Could you check a few things on this model? Use its own coordinates, in mm. A direction names the side the tool comes from. Give positions to 0.01 mm unless a question says otherwise; leave off trailing zeros. Order: outer loops, then holes, each group sorted by start corner. A loop starts at its lowest first (then second) coordinate and runs counter-clockwise, first axis right, second up.
(1) Imagine slicing it at C-C, the plane y = 37. Write out the boundary of the cut face in (x, z), then the cut area to 3 significant figures.
(2) If I drill on probe 1 along X at (y, z) = (2.7, 11.5); probe 2 along Y at (x, z) = (11, 6); probe 3 along Y at (x, z) = (-0.75, -5.5), over which ranges is the centre line in solid material (lowest first)?
(3) Imagine slicing it at A-A, the plane z = 0. Write out the boundary of the cut face in (x, y) (3 decimals), then the cut area to 3 significant figures.
(4) On a 3-axis mill with a long thin cutter (end or side, diameter ignored), from which of +Z, -Z, +X, -X, +Y, -Y can I reach the whole of each face in a straight line? I mean faces 5 (the flat face through (-11, 5, 12)), 6 (the flat face through (8.5, 30, -12)), 7 (the flat face through (-8.5, 30, 12)), 8 (the cylindrical face through (9.1, 30.06, 9.07)). Say none if no direction works.
(5) If we mould it in two halves opening along Z, with no side actions, what happens to faces 1 (the flat face through (-11, 5, -11)), 2 (the cylindrical face through (1.01, 14.28, 0.65)), 3 (the flat face through (14, 16, 0)), 4 (the flat face through (-12, 30, 8.5))? For each: released by +Z, released by -Z, zero draft, split by the parting line, or undercut.
(6) Imagine slicing it at B-B, the plane x = 0. Write out the boundary of the cut face in (y, z) (3 decimals), then the cut area to 3 significant figures.
(7) Will these pins go through, and if not, where does the flat tip stop? pin 1 (0.8 mm diameter, centred on y = 30, z = 12, fed in from +X); pin 2 (2.5 mm diameter, centred on x = -10, z = -11.5, fed in from +Y); pin 3 (5.5 mm diameter, centred on x = 10, z = 10, fed in from +Y).
(8) Imagine slicing it at D-D, the plane x = -4. Write out the boundary of the cut face in (y, z), then the cut area to 3 significant figures.
from build123d import *

# Parameters (mm, degrees)
SKETCH_1_W          = 28
SKETCH_1_H          = 28
EXTRUDE_1_DEPTH     = 31.8
SKETCH_2_R          = 10.975
EXTRUDE_2_DEPTH     = 2
SKETCH_3_R          = 2.5
EXTRUDE_3_DEPTH     = 18.2
EXTRUDE_START       = 16
SKETCH_4_R          = 2.5
EXTRUDE_4_DEPTH     = 16
FILLET_1_R          = 2
SKETCH_5_R          = 1.25
CUT_EXTRUDE_1_DEPTH = 5
CUT_EXTRUDE_2_DEPTH = 2.5
CHAMFER_1_SIZE      = 1
FILLET_2_R          = 0.5
SKETCH_7_R          = 1.2
CUT_EXTRUDE_3_DEPTH = 71.823724858


with BuildPart() as part:
    # 草图1 → 凸台-拉伸1 (new body)
    with BuildSketch(Plane(origin=(0, 0, 0), x_dir=(1, 0, 0), z_dir=(0, 1, 0))):
        Rectangle(SKETCH_1_W, SKETCH_1_H)
    extrude(amount=EXTRUDE_1_DEPTH)

    # 草图2 → 凸台-拉伸2 (add)
    with BuildSketch(Plane(origin=(0, 0, 0), x_dir=(-1, 0, 0), z_dir=(0, -1, 0))):
        with Locations(Location((0, 0, 0), (0, 0, 90))):
            Circle(SKETCH_2_R)
    extrude(amount=EXTRUDE_2_DEPTH)

    # 草图3 → 凸台-拉伸3 (add)
    with BuildSketch(Plane.XZ.offset(2)):
        with Locations(Location((0, 0, 0), (0, 0, 270))):
            Circle(SKETCH_3_R)
    extrude(amount=EXTRUDE_3_DEPTH)

    # 草图4 → 凸台-拉伸4 (add)
    with BuildSketch(Plane(origin=(0, 31.8, 0), x_dir=(1, 0, 0), z_dir=(0, 1, 0)).offset(EXTRUDE_START)):
        with Locations(Location((0, 0, 0), (0, 0, 90))):
            Circle(SKETCH_4_R)
    extrude(amount=-EXTRUDE_4_DEPTH)

    # 圆角1
    fillet_1_edges = [part.edges().sort_by_distance(p)[0] for p in [
        (-14, 15.9, -14),
        (14, 15.9, -14),
        (14, 15.9, 14),
        (-14, 15.9, 14),
    ]]
    fillet(fillet_1_edges, radius=FILLET_1_R)

    # 草图5 → 切除-拉伸1 (cut)
    with BuildSketch(Plane.XZ):
        with Locations(Location((-11.5, 11.5, 0), (0, 0, 270))):
            Circle(SKETCH_5_R)
        with Locations(Location((11.5, 11.5, 0), (0, 0, 270))):
            Circle(SKETCH_5_R)
        with Locations(Location((11.5, -11.5, 0), (0, 0, 270))):
            Circle(SKETCH_5_R)
        with Locations(Location((-11.5, -11.5, 0), (0, 0, 270))):
            Circle(SKETCH_5_R)
    extrude(amount=-CUT_EXTRUDE_1_DEPTH, mode=Mode.SUBTRACT)

    # 草图6 → 切除-拉伸2 (cut)
    with BuildSketch(Plane(origin=(0, 31.8, 0), x_dir=(1, 0, 0), z_dir=(0, 1, 0))):
        with BuildLine():
            Line((-14, -8.5), (-10.5, -8.5))
            ThreePointArc((-10.5, -8.5), (-9.085786438, -9.085786438), (-8.5, -10.5))
            Line((-8.5, -10.5), (-8.5, -14))
            Line((-8.5, -14), (-14, -14))
            Line((-14, -14), (-14, -8.5))
        make_face()
        with BuildLine():
            Line((14, 8.5), (10.5, 8.5))
            ThreePointArc((10.5, 8.5), (9.085786438, 9.085786438), (8.5, 10.5))
            Line((8.5, 10.5), (8.5, 14))
            Line((8.5, 14), (14, 14))
            Line((14, 14), (14, 8.5))
        make_face()
        with BuildLine():
            Line((-8.5, 14), (-14, 14))
            Line((-14, 14), (-14, 8.5))
            Line((-14, 8.5), (-10.5, 8.5))
            ThreePointArc((-10.5, 8.5), (-9.085786438, 9.085786438), (-8.5, 10.5))
            Line((-8.5, 10.5), (-8.5, 14))
        make_face()
        with BuildLine():
            Line((14, -8.5), (10.5, -8.5))
            ThreePointArc((10.5, -8.5), (9.085786438, -9.085786438), (8.5, -10.5))
            Line((8.5, -10.5), (8.5, -14))
            Line((8.5, -14), (14, -14))
            Line((14, -14), (14, -8.5))
        make_face()
    extrude(amount=-CUT_EXTRUDE_2_DEPTH, mode=Mode.SUBTRACT)

    # 倒角1
    chamfer_1_edges = [part.edges().sort_by_distance(p)[0] for p in [
        (-12.25, 31.8, -8.5),
        (-9.085786438, 31.8, -9.085786438),
        (-8.5, 31.8, -12.25),
        (8.5, 31.8, -12.25),
        (9.085786438, 31.8, -9.085786438),
        (12.25, 31.8, -8.5),
        (-8.5, 31.8, 12.25),
        (-9.085786438, 31.8, 9.085786438),
        (-12.25, 31.8, 8.5),
        (12.25, 31.8, 8.5),
        (9.085786438, 31.8, 9.085786438),
        (8.5, 31.8, 12.25),
    ]]
    chamfer(chamfer_1_edges, length=CHAMFER_1_SIZE)

    # 圆角2
    fillet_2_edges = [part.edges().sort_by_distance(p)[0] for p in [
        (-10.25, 29.3, -14),
        (-8.5, 30.05, -14),
        (-14, 29.3, -10.25),
        (-14, 30.05, -8.5),
        (14, 29.3, -10.25),
        (14, 30.05, -8.5),
        (10.25, 29.3, -14),
        (8.5, 30.05, -14),
        (-14, 29.3, 10.25),
        (-14, 30.05, 8.5),
        (-10.25, 29.3, 14),
        (-8.5, 30.05, 14),
        (14, 31.8, 0),
        (0, 31.8, -14),
        (-14, 31.8, 0),
        (0, 31.8, 14),
        (-7.5, 31.8, -12.25),
        (-8.378679656, 31.8, -8.378679656),
        (-12.25, 31.8, -7.5),
        (-8.378679656, 31.8, 8.378679656),
        (-12.25, 31.8, 7.5),
        (-7.5, 31.8, 12.25),
        (8.378679656, 31.8, -8.378679656),
        (12.25, 31.8, -7.5),
        (7.5, 31.8, -12.25),
        (8.378679656, 31.8, 8.378679656),
        (7.5, 31.8, 12.25),
        (12.25, 31.8, 7.5),
        (14, 31.3, -8),
        (14, 31.3, 8),
        (-8, 31.3, 14),
        (8, 31.3, 14),
        (-8, 31.3, -14),
        (8, 31.3, -14),
        (-14, 31.3, -8),
        (-14, 31.3, 8),
        (0, 31.8, 2.5),
        (0, 0, -14),
        (-14, 0, 0),
        (14, 0, 0),
        (0, 0, 14),
        (-13.414213562, 0, 13.414213562),
        (-13.414213562, 0, -13.414213562),
        (13.414213562, 0, 13.414213562),
        (13.414213562, 0, -13.414213562),
        (-13.414213562, 29.3, 13.414213562),
        (-13.414213562, 29.3, -13.414213562),
        (13.414213562, 29.3, 13.414213562),
        (13.414213562, 29.3, -13.414213562),
        (10.25, 29.3, 14),
        (14, 29.3, 10.25),
        (14, 30.05, 8.5),
        (8.5, 30.05, 14),
    ]]
    fillet(fillet_2_edges, radius=FILLET_2_R)

    # 草图7 → 切除-拉伸3 (cut, through all)
    with BuildSketch(Plane(origin=(0, 47.8, 0), x_dir=(1, 0, 0), z_dir=(0, 1, 0))):
        with Locations(Location((0, 0, 0), (0, 0, 270))):
            Circle(SKETCH_7_R)
    extrude(amount=-CUT_EXTRUDE_3_DEPTH, mode=Mode.SUBTRACT)


solid = part.part
Answer block:
1. outline: circle Ø5 at (0, 0); hole circle Ø2.4 at (0, 0)
1. area: 15.1 mm2
2. probe 1: x = -14 to -12.75, -10.25 to 10.25, 12.75 to 14
2. probe 2: y = 0 to 31.8
2. probe 3: y = -2 to 31.8
3. outline: (-14, 0.5) arc R0.5 ccw to (-13.5, 0) - (-10.975, 0) - (-10.975, -2) - (-2.5, -2) - (-2.5, -20.2) - (-1.2, -20.2) - (-1.2, 47.8) - (-2.5, 47.8) - (-2.5, 32.3) arc R0.5 cw to (-3, 31.8) - (-13.5, 31.8) arc R0.5 ccw to (-14, 31.3) - close; (1.2, -20.2) - (2.5, -20.2) - (2.5, -2) - (10.975, -2) - (10.975, 0) - (13.5, 0) arc R0.5 ccw to (14, 0.5) - (14, 31.3) arc R0.5 ccw to (13.5, 31.8) - (3, 31.8) arc R0.5 cw to (2.5, 32.3) - (2.5, 47.8) - (1.2, 47.8) - close
3. area: 942 mm2
4. face 5: -Y
4. face 6: -Z, +X, +Y
4. face 7: +Z, -X, +Y
4. face 8: +Z, +X, +Y
5. face 1: undercut
5. face 2: undercut
5. face 3: zero draft
5. face 4: released by +Z
6. outline: (-20.2, -2.5) - (-2, -2.5) - (-2, -10.975) - (0, -10.975) - (0, -13.5) arc R0.5 ccw to (0.5, -14) - (31.3, -14) arc R0.5 ccw to (31.8, -13.5) - (31.8, -3) arc R0.5 cw to (32.3, -2.5) - (47.8, -2.5) - (47.8, -1.2) - (-20.2, -1.2) - close; (-20.2, 1.2) - (47.8, 1.2) - (47.8, 2.5) - (32.3, 2.5) arc R0.5 cw to (31.8, 3) - (31.8, 13.5) arc R0.5 ccw to (31.3, 14) - (0.5, 14) arc R0.5 ccw to (0, 13.5) - (0, 10.975) - (-2, 10.975) - (-2, 2.5) - (-20.2, 2.5) - close
6. area: 942 mm2
7. pin 1: stops at x = 8.5
7. pin 2: stops at y = 29.3
7. pin 3: stops at y = 31.8
8. outline: (-2, -10.22) - (0, -10.22) - (0, -13.5) arc R0.5 ccw to (0.5, -14) - (31.3, -14) arc R0.5 ccw to (31.8, -13.5) - (31.8, 13.5) arc R0.5 ccw to (31.3, 14) - (0.5, 14) arc R0.5 ccw to (0, 13.5) - (0, 10.22) - (-2, 10.22) - close
8. area: 931 mm2
